Answer from the drawing. Dimensions are ordinates in mm from the lowest x, y and z of the part. A direction names the side the tool comes from. Give positions to 0.01 mm unless a question says otherwise; leave off trailing zeros. Write each loop counter-clockwise with the first axis right and the second up, starting at its lowest first coordinate (ties: lowest second). Pieces come first, ordered by that corner, then holes. Notation, with made-up numbers: M 25.5,-13 L 80.5,-13 A27 cw 80.5,15 Z; hole C -15.5,42 d3. An arc over 180 degrees is marked long. Put each result on its own line as item: value.
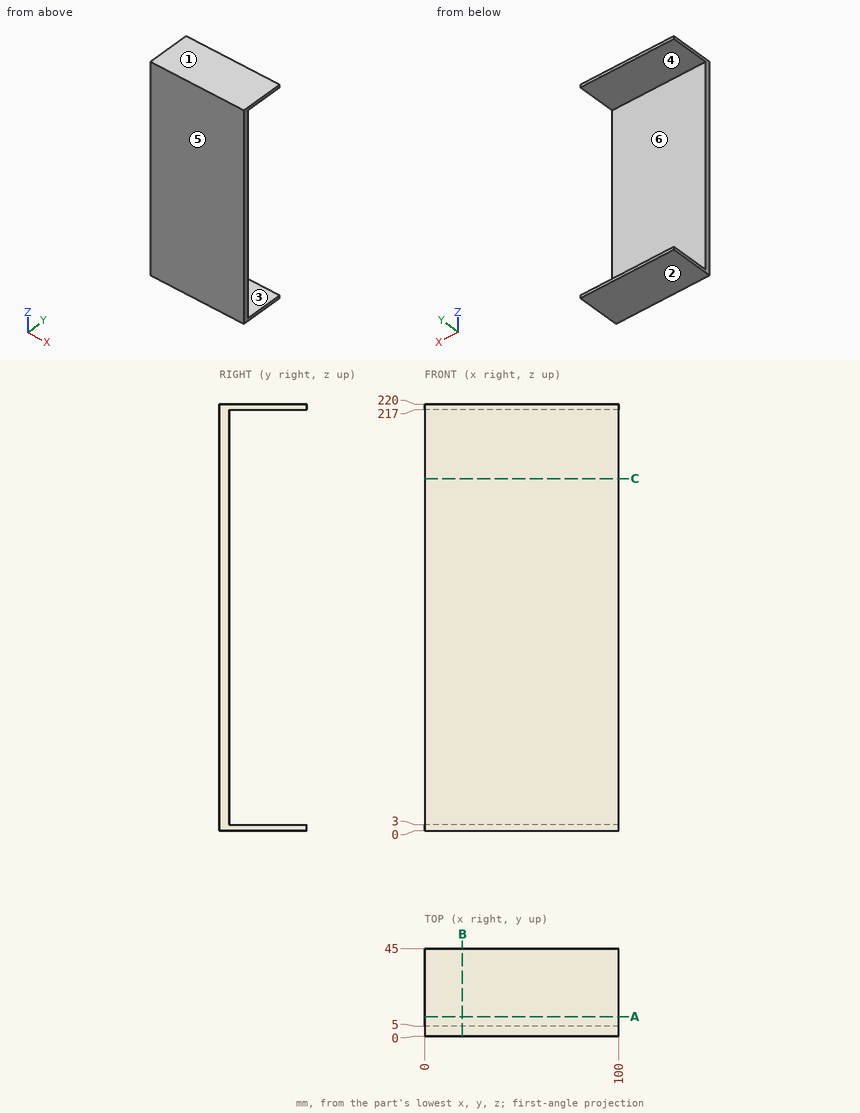
(1) Section C-C on z = 181.5 is taken. Determine the outline of the cut face in (x, y), and give its area (3 significant figures).
Result:
outline: M 0,0 L 100,0 L 100,5 L 0,5 Z
area: 500 mm²
(2) Straight lines are drawn through the part: line 1 along Z through (x, y) = (27, 30.5); line 2 along Y through (x, z) = (15.5, 131). For each, find the intervals that lie inside material, in ascending order. Write a range as from..to.
Result:
line 1: z = 0..3, 217..220
line 2: y = 0..5
(3) For a pull along Z with two mould halves and no side action, classify the marked faces 1, 2, 3 and 4 as +Z half, -Z half, draft (parallel to the pull), parting line (faces both ways), or undercut.
Result:
face 1: +Z half
face 2: -Z half
face 3: undercut
face 4: undercut
(4) Given pin 1 Ø2 at (x, z) = (38, 44) entering from +Y, flat-ended and moving along its own axis, determine where the tip first touches the part or whether it passes through.
Result:
pin 1: stops at y = 5
(5) Which of the six approach directions +Z, -Z, +X, -X, +Y, -Y give full straight-line access (tool end or side, diameter ignored) to the marked faces 5 and 6?
Result:
face 5: +Z, -Z, +X, -X, -Y
face 6: +X, -X, +Y
(6) Section A-A on y = 10 is taken. Determine the outline of the cut face in (x, z), and give its area (3 significant figures).
Result:
outline: M 0,0 L 100,0 L 100,3 L 0,3 Z; M 0,217 L 100,217 L 100,220 L 0,220 Z
area: 600 mm²
(7) Section B-B on x = 19.5 is taken. Determine the outline of the cut face in (y, z).
Result:
outline: M 0,0 L 45,0 L 45,3 L 5,3 L 5,217 L 45,217 L 45,220 L 0,220 Z
